Build history of the part. All positions in model axes, mm. A direction names the side the tool comes from. Coordinates: 2 decimals unless noted, no trailing zeros. Order: outer loops, then holes, each group sorted by start corner. A loop starts at its lowest first (then second) coordinate and runs counter-clockwise, first axis right, second up. Notation, with made-up numbers: (15.5, -5) - (61.5, -5) arc R18 ccw to (61.5, 7) - close; hole circle Ø7 at (16.25, 76.25). An arc over 180 degrees is marked (long way). Return JSON: item names as keys, results as strings.
from build123d import *

# Parameters (mm, degrees)
BOSS_EXTRUDE1_DEPTH = 10
BOSS_EXTRUDE2_DEPTH = 5


with BuildPart() as part:
    # Sketch1 → Boss-Extrude1 (new, symmetric)
    with BuildSketch(Plane.XY):
        with BuildLine():
            Line((23.096988313, 9.567085809), (55.432771951, 22.961005942))
            ThreePointArc((55.432771951, 22.961005942), (42.426406871, 42.426406871), (22.961005942, 55.432771951))
            ThreePointArc((22.961005942, 55.432771951), (0, 60), (-22.961005942, 55.432771951))
            ThreePointArc((-22.961005942, 55.432771951), (-42.426406871, 42.426406871), (-55.432771951, 22.961005942))
            Line((-55.432771951, 22.961005942), (-23.096988313, 9.567085809))
            ThreePointArc((-23.096988313, 9.567085809), (0, 25), (23.096988313, 9.567085809))
        make_face()
        with BuildLine():
            Line((-69.290964938, 28.701257427), (-55.432771951, 22.961005942))
            ThreePointArc((-55.432771951, 22.961005942), (-42.426406871, 42.426406871), (-22.961005942, 55.432771951))
            Line((-22.961005942, 55.432771951), (-28.701257427, 69.290964938))
            ThreePointArc((-28.701257427, 69.290964938), (-53.033008589, 53.033008589), (-69.290964938, 28.701257427))
        make_face()
        with BuildLine():
            Line((55.432771951, 22.961005942), (69.290964938, 28.701257427))
            ThreePointArc((69.290964938, 28.701257427), (53.033008589, 53.033008589), (28.701257427, 69.290964938))
            Line((28.701257427, 69.290964938), (22.961005942, 55.432771951))
            ThreePointArc((22.961005942, 55.432771951), (42.426406871, 42.426406871), (55.432771951, 22.961005942))
        make_face()
        with BuildLine():
            ThreePointArc((-22.961005942, -55.432771951), (-42.426406871, -42.426406871), (-55.432771951, -22.961005942))
            Line((-55.432771951, -22.961005942), (-69.290964938, -28.701257427))
            ThreePointArc((-69.290964938, -28.701257427), (-53.033008589, -53.033008589), (-28.701257427, -69.290964938))
            Line((-28.701257427, -69.290964938), (-22.961005942, -55.432771951))
        make_face()
        with BuildLine():
            Line((55.432771951, -22.961005942), (23.096988313, -9.567085809))
            ThreePointArc((23.096988313, -9.567085809), (0, -25), (-23.096988313, -9.567085809))
            Line((-23.096988313, -9.567085809), (-55.432771951, -22.961005942))
            ThreePointArc((-55.432771951, -22.961005942), (-42.426406871, -42.426406871), (-22.961005942, -55.432771951))
            ThreePointArc((-22.961005942, -55.432771951), (0, -60), (22.961005942, -55.432771951))
            ThreePointArc((22.961005942, -55.432771951), (42.426406871, -42.426406871), (55.432771951, -22.961005942))
        make_face()
        with BuildLine():
            Line((69.290964938, -28.701257427), (55.432771951, -22.961005942))
            ThreePointArc((55.432771951, -22.961005942), (42.426406871, -42.426406871), (22.961005942, -55.432771951))
            Line((22.961005942, -55.432771951), (28.701257427, -69.290964938))
            ThreePointArc((28.701257427, -69.290964938), (53.033008589, -53.033008589), (69.290964938, -28.701257427))
        make_face()
    extrude(amount=BOSS_EXTRUDE1_DEPTH, both=True)

    # Sketch1_3 → Boss-Extrude2 (add, symmetric)
    with BuildSketch(Plane.XY):
        with BuildLine():
            ThreePointArc((-23.096988313, -9.567085809), (0, -25), (23.096988313, -9.567085809))
            Line((23.096988313, -9.567085809), (55.432771951, -22.961005942))
            ThreePointArc((55.432771951, -22.961005942), (58.847116824, -11.705419321), (60, 0))
            ThreePointArc((60, 0), (58.847116824, 11.705419321), (55.432771951, 22.961005942))
            Line((55.432771951, 22.961005942), (23.096988313, 9.567085809))
            ThreePointArc((23.096988313, 9.567085809), (0, 25), (-23.096988313, 9.567085809))
            Line((-23.096988313, 9.567085809), (-55.432771951, 22.961005942))
            ThreePointArc((-55.432771951, 22.961005942), (-60, 0), (-55.432771951, -22.961005942))
            Line((-55.432771951, -22.961005942), (-23.096988313, -9.567085809))
        make_face()
    extrude(amount=BOSS_EXTRUDE2_DEPTH, both=True)


solid = part.part
1. Mould opens along Y. For faces 1 (the cylindrical face through (0, -25, -7)), 2 (the cylindrical face through (0, -60, 0)), 3 (the cylindrical face through (53.324, 52.741, -0.14)) say: pulls with the +Y half, pulls with the -Y half, needs draft (parallel to the pull), parting line crosses it, or undercut.
Check values:
{"face 1": "undercut", "face 2": "pulls with the -Y half", "face 3": "pulls with the +Y half"}
2. Cut at B-B on y = 17. Give the cut face in (x, z).
Check values:
{"outline": "(-57.54, -5) - (-41.04, -5) - (-41.04, -10) - (-18.33, -10) - (-18.33, -5) - (18.33, -5) - (18.33, -10) - (41.04, -10) - (41.04, -5) - (57.54, -5) - (57.54, 5) - (41.04, 5) - (41.04, 10) - (18.33, 10) - (18.33, 5) - (-18.33, 5) - (-18.33, 10) - (-41.04, 10) - (-41.04, 5) - (-57.54, 5) - close"}
3. Cut at C-C on x = -15.5. Give the cut face in (y, z), plus the area to 3 significant figures.
Check values:
{"outline": "(-57.96, -10) - (-19.62, -10) - (-19.62, -5) - (19.62, -5) - (19.62, -10) - (57.96, -10) - (57.96, 10) - (19.62, 10) - (19.62, 5) - (-19.62, 5) - (-19.62, 10) - (-57.96, 10) - close", "area": "1,930 mm²"}
4. Tool access for faces 4 (the flat face through (-1, 0, -5)), 5 (the cylindrical face through (-60, 0, 0)), 6 (the flat face through (25.79, -62.26, 0.14)), 7 (the cylindrical face through (0, -25, 8)), 8 (the flat face through (25.87, 62.46, -0.14)): list every direction of +Z, -Z, +X, -X, +Y, -Y with a clear straight run to the whole face (end or side of a thin tool).
Check values:
{"face 4": "-Z", "face 5": "+Z, -Z, -X", "face 6": "+Z, -Z, -Y", "face 7": "+Z", "face 8": "+Z, -Z, +Y"}
5. Cut at D-D on x = -32.5. Give the cut face in (y, z).
Check values:
{"outline": "(-67.59, -10) - (-13.46, -10) - (-13.46, -5) - (13.46, -5) - (13.46, -10) - (67.59, -10) - (67.59, 10) - (13.46, 10) - (13.46, 5) - (-13.46, 5) - (-13.46, 10) - (-67.59, 10) - close"}
6. Probe L1, parallel to Y at x = -1, z = -9; L2, parallel to Z at x = -38, y = 1.5; L3, parallel to X at y = -21.5, z = 7.75. List the from-to ranges inside material, lowest first.
Check values:
{"L1": "-59.99 to -24.98, 24.98 to 59.99", "L2": "-5 to 5", "L3": "-51.91 to -12.76, 12.76 to 51.91"}
7. Drop flat-ended pins along their axis: pin 1 (12 mm diameter, centred on y = 54, z = -5.5, fed in from -X); pin 2 (1.5 mm diameter, centred on y = 22.5, z = -6.5, fed in from -X); pin 3 (3 mm diameter, centred on y = 16, z = -7.5, fed in from +X). Give the stop position or say it passes through.
Check values:
{"pin 1": "x = -57.63", "pin 2": "x = -56.13", "pin 3": "x = 42.25"}
8. Cut at A-A on z = -7. Give the cut face in (x, y), plus the area to 3 significant figures.
Check values:
{"outline": "(-69.29, -28.7) arc R75 ccw to (-28.7, -69.29) - (-22.96, -55.43) arc R60 ccw to (22.96, -55.43) - (28.7, -69.29) arc R75 ccw to (69.29, -28.7) - (23.1, -9.57) arc R25 cw to (-23.1, -9.57) - close; (-69.29, 28.7) - (-23.1, 9.57) arc R25 cw to (23.1, 9.57) - (69.29, 28.7) arc R75 ccw to (28.7, 69.29) - (22.96, 55.43) arc R60 ccw to (-22.96, 55.43) - (-28.7, 69.29) arc R75 ccw to start", "area": "10,200 mm²"}
